Here's how the part is built. I have some questions about the finished solid (model axes, mm). A direction names the side the tool comes from. Coordinates: 2 decimals unless noted, no trailing zeros. Write each loop counter-clockwise with the first axis right and the second up, starting at its lowest first coordinate (ties: lowest second). Pieces come first, ordered by that corner, then holes.
Item 1: I want a section at B-B (z = 0). Please give me the cut outline in (x, y), and give its area (3 significant figures).
Item 2: I want a section at A-A (x = 0). Please give me the cut outline in (y, z), and give its area (3 significant figures).
Item 3: I want a section at C-C (y = 60.5). Please give me the cut outline in (x, z), and give its area (3 significant figures).
Item 4: I'm going to push flat-ended pins straight in: P1, Ø2.5, axis at x = 8, z = -14, coming from the -Y side; P2, Ø2, axis at x = 4, y = 32.5, coming from the -Z side; P3, Ø12, axis at x = 4, y = -2.5, coming from the +Z side. Where does each tip first touch, or does it pass through?
Item 5: I want a section at D-D (x = -12). Please give me the cut outline in (y, z), and give its area (3 significant figures).
Item 6: Please list where these lines run through material, in increasing order: line 1 (Z direction, x = -7.75, y = 1.8); line 2 (Z direction, x = 7, y = 1); line 3 (Y direction, x = -9.5, z = -11).
Item 7: For faces 4 (the face through (-3, -6.5, -8)), 5 (the face through (-15.4, 52.7, -7.7)), 6 (the face through (-14.6, 10.8, -11.2)), which set-ups out of +Z, -Z, +X, -X, +Y, -Y let a thin tool reach every point of the face, with its end or its side?
Item 8: If we mould it in two halves opening along X, with no side actions, what happens to faces 1 (the face through (3.772, 37.135, -16.986)), 2 (the face through (8, 4, 13)), 3 (the face through (14, 22, 11))? For each: pulls with the +X half, pulls with the -X half, needs draft (parallel to the pull), parting line crosses it, or undercut.
from build123d import *

# Parameters (mm, degrees)
F0_R      = 18.4
F1_DEPTH  = 22
F2_R      = 17.4
F3_DEPTH  = 30.7
F4_R      = 17
F5_DEPTH  = 15.4
F6_R      = 6
F7_DEPTH  = 6.5
F8_R      = 3
F9_DEPTH  = 15.5
F10_R     = 1.5
F11_DEPTH = 4


with BuildPart() as f1:
    # F0 (on Front) → F1 (new body)
    with BuildSketch(Plane.XZ):
        Circle(F0_R)
    extrude(amount=-F1_DEPTH)

    # F2 (on face) → F3 (join)
    with BuildSketch(Plane(origin=(0, 22, 0), x_dir=(-1, 0, 0), z_dir=(0, 1, 0))):
        Circle(F2_R)
    extrude(amount=F3_DEPTH)

    # F4 (on face) → F5 (join)
    with BuildSketch(Plane(origin=(0, 52.7, 0), x_dir=(-1, 0, 0), z_dir=(0, 1, 0))):
        Circle(F4_R)
    extrude(amount=F5_DEPTH)

    # F6 (on face) → F7 (join)
    with BuildSketch(Plane.XZ):
        with Locations((0, -7)):
            Circle(F6_R)
    extrude(amount=F7_DEPTH)

    # F8 (on face) → F9 (join)
    with BuildSketch(Plane.XZ.offset(6.5)):
        with Locations((0, -7)):
            Circle(F8_R)
    extrude(amount=F9_DEPTH)

    # F10 (on face) → F11 (cut)
    with BuildSketch(Plane.XZ):
        with Locations((-15.5, 0)):
            Circle(F10_R)
        with Locations((-7.75, 13.423394)):
            Circle(F10_R)
        with Locations((7.75, 13.423394)):
            Circle(F10_R)
        with Locations((15.5, 0)):
            Circle(F10_R)
        with Locations((-7.75, -13.423394)):
            Circle(F10_R)
        with Locations((7.75, -13.423394)):
            Circle(F10_R)
    extrude(amount=-F11_DEPTH, mode=Mode.SUBTRACT)


solid = f1.part
Answer:
1. outline: (-18.4, 0) - (-17, 0) - (-17, 4) - (-14, 4) - (-14, 0) - (14, 0) - (14, 4) - (17, 4) - (17, 0) - (18.4, 0) - (18.4, 22) - (17.4, 22) - (17.4, 52.7) - (17, 52.7) - (17, 68.1) - (-17, 68.1) - (-17, 52.7) - (-17.4, 52.7) - (-17.4, 22) - (-18.4, 22) - close
1. area: 2,380 mm2
2. outline: (-22, -10) - (-6.5, -10) - (-6.5, -13) - (0, -13) - (0, -18.4) - (22, -18.4) - (22, -17.4) - (52.7, -17.4) - (52.7, -17) - (68.1, -17) - (68.1, 17) - (52.7, 17) - (52.7, 17.4) - (22, 17.4) - (22, 18.4) - (0, 18.4) - (0, -1) - (-6.5, -1) - (-6.5, -4) - (-22, -4) - close
2. area: 2,570 mm2
3. outline: circle Ø34 at (0, 0)
3. area: 908 mm2
4. P1: stops at y = 0
4. P2: stops at z = -17.14
4. P3: stops at z = 18.4
5. outline: (0, -13.95) - (22, -13.95) - (22, -12.6) - (52.7, -12.6) - (52.7, -12.04) - (68.1, -12.04) - (68.1, 12.04) - (52.7, 12.04) - (52.7, 12.6) - (22, 12.6) - (22, 13.95) - (0, 13.95) - close
5. area: 1,760 mm2
6. line 1: z = -16.69 to -14.92, -11.92 to 11.92, 14.92 to 16.69
6. line 2: z = -17.02 to -14.72, -12.12 to 12.12, 14.72 to 17.02
6. line 3: y = 0 to 68.1
7. face 4: -Y
7. face 5: +Y
7. face 6: +Y, -Y
8. face 1: parting line crosses it
8. face 2: undercut
8. face 3: needs draft
